Model file for the job. Use its own axes, mm. A direction names the side the tool comes from. Coordinates: 2 decimals unless noted, no trailing zeros. Order: outer loops, then holes, each group sorted by start corner. A loop starts at its lowest first (then second) coordinate and runs counter-clockwise, first axis right, second up. Notation, with made-up numbers: (25.25, 4) -> (72.25, 4) arc R28 cw to (72.25, 31) -> close; hole circle Ø3 at (29.5, 76.25). An arc over 180 degrees is marked (long way). Write item = value, one per line. Start each with the question number.
Q1. 3-axis set-ups, long thin cutter, end or side, ignore diameter. For faces 4 (the face through (2.7, -4, 0)), 5 (the face through (-1.2, -22, -0.9)), 6 (the face through (7, -15, -0.6)), 7 (the face through (1.797, -14.902, -0.998)): which of +Z, -Z, +X, -X, +Y, -Y reach the whole face in a straight line?
Q2. Flat gauge pins, fed straight in: pin 1 (1 mm diameter, centred on y = -5.5, z = 0, fed in from -X); pin 2 (4.5 mm diameter, centred on x = 8, y = -23, fed in from -Z); pin 3 (1 mm diameter, centred on y = -19.5, z = -3, fed in from -X). Where does each tip first touch, or does it go through?
Q3. Cut at A-A, the plane z = -2.1. List the corners of the cut face in (x, y), plus the area to 3 significant figures.
Q4. Mould opens along X. For faces 1 (the face through (9, 0, 0)), 2 (the face through (15, -15, 0)), 3 (the face through (8.37, -8.66, -0.01)) say: +X half, -X half, draft (parallel to the pull), parting line (faces both ways), or undercut.
Q5. Cut at B-B, the plane x = 8. List the corners of the cut face in (y, z).
Q6. Cut at D-D, the plane y = -12.5. List the corners of the cut face in (x, z).
Q7. Wall check: line 1 (X direction, y = -15, z = -2.1); line 2 (Y direction, x = 8, z = 0.25); line 3 (Z direction, x = 12, y = -1.5). Give the ranges that are in metal, low to high. Write a range as from..to.
Q8. Cut at C-C, the plane y = -7. List the corners of the cut face in (x, z).
from build123d import *

# Parameters (mm, degrees)
Y_KSEKLIK_EKSTR_ZYON1_DEPTH = 30
KES_EKSTR_ZYON2_START       = -8
KES_EKSTR_ZYON2_DEPTH       = 8
IZIM4_R                     = 1.7
KES_EKSTR_ZYON3_DEPTH       = 1.2


with BuildPart() as part:
    # Çizim1 → Yükseklik-Ekstrüzyon1 (new body)
    with BuildSketch(Plane(origin=(0, 0, 0), x_dir=(1, 0, 0), z_dir=(0, 1, 0))):
        with BuildLine():
            Line((0, 0.6), (15, 0.6))
            Line((15, 0.6), (15, -0.6))
            Line((15, -0.6), (0, -0.6))
            ThreePointArc((0, -0.6), (-1.319038138, 4.455873169), (2.301841896, 0.688786378))
            Line((2.301841896, 0.688786378), (1.278801053, 1.315992432))
            ThreePointArc((1.278801053, 1.315992432), (-0.732798966, 3.408818427), (0, 0.6))
        make_face()
    extrude(amount=-Y_KSEKLIK_EKSTR_ZYON1_DEPTH)

    # Çizim3 → Kes-Ekstrüzyon2 (cut)
    with BuildSketch(Plane.XZ.offset(30).offset(KES_EKSTR_ZYON2_START)):
        with BuildLine():
            Line((1.278801053, -1.315992432), (2.301841896, -0.688786378))
            ThreePointArc((2.301841896, -0.688786378), (-1.319038138, -4.455873169), (0, 0.6))
            Line((0, 0.6), (2.7, 0.6))
            Line((2.7, 0.6), (2.7, -0.6))
            Line((2.7, -0.6), (0, -0.6))
            ThreePointArc((0, -0.6), (-0.732798966, -3.408818427), (1.278801053, -1.315992432))
        make_face()
    kes_ekstr_zyon2 = extrude(amount=KES_EKSTR_ZYON2_DEPTH, mode=Mode.SUBTRACT)

    # Çizim4 → Kes-Ekstrüzyon3 (cut)
    with BuildSketch(Plane(origin=(0, 0, -0.6), x_dir=(-1, 0, 0), z_dir=(0, 0, -1))):
        with Locations((-8, -23)):
            Circle(IZIM4_R)
        with Locations((-8, -7)):
            Circle(IZIM4_R)
    extrude(amount=-KES_EKSTR_ZYON3_DEPTH, mode=Mode.SUBTRACT)

    # Aynalama1: Kes-Ekstrüzyon2 across plane
    add(kes_ekstr_zyon2.mirror(Plane(origin=(0, -15, 0), x_dir=(0, 0, 1), z_dir=(0, -1, 0))), mode=Mode.SUBTRACT)


solid = part.part
Here are the results:
q1.face_4 = +Z, -Z, -X, +Y
q1.face_5 = +Z, -Z, -X, -Y
q1.face_6 = +X, +Y, -Y
q1.face_7 = +Y, -Y
q2.pin_1 = 2.7
q2.pin_2 = -0.6
q2.pin_3 = -2.67
q3.outline = (-2.7, -22) -> (-1.5, -22) -> (-1.5, -8) -> (-2.7, -8) -> close; (1.5, -22) -> (2.7, -22) -> (2.7, -8) -> (1.5, -8) -> close
q3.area = 33.6 mm²
q4.face_1 = draft
q4.face_2 = +X half
q4.face_3 = undercut
q5.outline = (-30, -0.6) -> (-24.7, -0.6) -> (-24.7, 0.6) -> (-30, 0.6) -> close; (-21.3, -0.6) -> (-8.7, -0.6) -> (-8.7, 0.6) -> (-21.3, 0.6) -> close; (-5.3, -0.6) -> (0, -0.6) -> (0, 0.6) -> (-5.3, 0.6) -> close
q6.outline = (0, -0.6) -> (15, -0.6) -> (15, 0.6) -> (0, 0.6) arc R2.7 ccw (long way) to (2.3, -0.69) -> (1.28, -1.32) arc R1.5 cw (long way) to start
q7.line_1 = -2.7..-1.5, 1.5..2.7
q7.line_2 = -30..-24.7, -21.3..-8.7, -5.3..0
q7.line_3 = -0.6..0.6
q8.outline = (2.7, -0.6) -> (6.3, -0.6) -> (6.3, 0.6) -> (2.7, 0.6) -> close; (9.7, -0.6) -> (15, -0.6) -> (15, 0.6) -> (9.7, 0.6) -> close
